```python
from build123d import *

# Parameters (mm, degrees)
SKETCH1_W                  = 100
SKETCH1_H                  = 196.50497
BASE_FLANGE1_DEPTH         = 2.54
CUT_EXTRUDE1_DEPTH         = 221.500917991
CUT_EXTRUDE1_DEPTH_BACK    = 221.500917991
SKETCH1_4_R                = 1.13
SKETCHED_START             = -70.001308696
SKETCHED_BEND3_OUTLINE_R   = 1.13
SKETCHED_BEND3_DEPTH       = 55.325410031
SKETCHED_BEND3_2_DEPTH     = 100
SKETCHED_BEND3_3_DEPTH     = 100
SKETCHED_START_2           = -123
SKETCHED_BEND3_4_OUTLINE_R = 1.13
SKETCHED_BEND3_4_DEPTH     = 4
CUT_EXTRUDE3_DEPTH         = 253.225301809
CUT_EXTRUDE3_DEPTH_BACK    = 253.225301809
SKETCH19_R                 = 1.725
F_4_40_TAPPED_HOLE1_D      = 2.2606


with BuildPart() as part:
    # Base-Flange1: sheet metal written as solids
    # Sketch1 → Base-Flange1 (new body)
    with BuildSketch(Plane.XY):
        with Locations((50, -98.252485)):
            Rectangle(SKETCH1_W, SKETCH1_H)
    extrude(amount=-BASE_FLANGE1_DEPTH)

    # Sketch1<4> → Cut-Extrude1 (cut, two sides: drawn at the far end of the back side and taken through both)
    with BuildSketch(Plane.XY.offset(-CUT_EXTRUDE1_DEPTH_BACK)):
        with Locations((11.9, -6.4268)):
            Circle(SKETCH1_4_R)
        with Locations((88.1, -6.4268)):
            Circle(SKETCH1_4_R)
        with Locations((88.1, -95.3268)):
            Circle(SKETCH1_4_R)
        with Locations((11.9, -95.3268)):
            Circle(SKETCH1_4_R)
    extrude(amount=CUT_EXTRUDE1_DEPTH + CUT_EXTRUDE1_DEPTH_BACK, mode=Mode.SUBTRACT)

    # Sketched Bend3: read off the stored shape, not the designer's step
    # Sketched Bend3 outline → Sketched Bend3 (cut)
    with BuildSketch(Plane(origin=(0, 0, 0), x_dir=(1, 0, 0), z_dir=(0, 0.707106781186549, 0.707106781186546)).offset(SKETCHED_START)):
        with Locations((88.1, -44.309515504)):
            Circle(SKETCHED_BEND3_OUTLINE_R)
        with Locations((11.9, -44.309515504)):
            Circle(SKETCHED_BEND3_OUTLINE_R)
    extrude(amount=SKETCHED_BEND3_DEPTH, mode=Mode.SUBTRACT)

    # Sketched Bend3 2 outline → Sketched Bend3 2 (cut)
    with BuildSketch(Plane.YZ):
        with BuildLine():
            ThreePointArc((-171.665649191, 0), (-169.42029242, -0.446629231), (-167.516770864, -1.718521672))
            Line((-167.516770864, -1.718521672), (-166.695292536, -2.54))
            Line((-166.695292536, -2.54), (0, -2.54))
            Line((0, -2.54), (0, 0))
            Line((0, 0), (-171.665649191, 0))
        make_face()
    extrude(amount=SKETCHED_BEND3_2_DEPTH, mode=Mode.SUBTRACT)

    # Sketched Bend3 3 outline → Sketched Bend3 3 (add)
    with BuildSketch(Plane.YZ):
        with BuildLine():
            Line((-48.542978443, -120.692314093), (-166.695292536, -2.54))
            Line((-166.695292536, -2.54), (-171.665649191, -2.54))
            ThreePointArc((-171.665649191, -2.54), (-170.392308339, -2.793283244), (-169.312822088, -3.514572896))
            Line((-169.312822088, -3.514572896), (-50.339029667, -122.488365317))
            Line((-50.339029667, -122.488365317), (-48.542978443, -120.692314093))
        make_face()
    extrude(amount=SKETCHED_BEND3_3_DEPTH)

    # Sketched Bend3 4 outline → Sketched Bend3 4 (cut)
    with BuildSketch(Plane(origin=(0, 0, 0), x_dir=(1, 0, 0), z_dir=(0, 0.707106781186549, 0.707106781186546)).offset(SKETCHED_START_2)):
        with Locations((11.9, 44.590484496)):
            Circle(SKETCHED_BEND3_4_OUTLINE_R)
        with Locations((88.1, 44.590484496)):
            Circle(SKETCHED_BEND3_4_OUTLINE_R)
        with Locations((88.1, -44.309515504)):
            Circle(SKETCHED_BEND3_4_OUTLINE_R)
        with Locations((11.9, -44.309515504)):
            Circle(SKETCHED_BEND3_4_OUTLINE_R)
    extrude(amount=SKETCHED_BEND3_4_DEPTH, mode=Mode.SUBTRACT)

    # Sketch19 → Cut-Extrude3 (cut, two sides: drawn at the far end of the back side and taken through both)
    with BuildSketch(Plane.XY.offset(-CUT_EXTRUDE3_DEPTH_BACK)):
        with Locations((10, -179.08497)):
            Circle(SKETCH19_R)
        with Locations((50, -179.08497)):
            Circle(SKETCH19_R)
        with Locations((90, -179.08497)):
            Circle(SKETCH19_R)
        with Locations((50, -189.08497)):
            Circle(SKETCH19_R)
        with Locations((90, -189.08497)):
            Circle(SKETCH19_R)
        with Locations((10, -189.08497)):
            Circle(SKETCH19_R)
    extrude(amount=CUT_EXTRUDE3_DEPTH + CUT_EXTRUDE3_DEPTH_BACK, mode=Mode.SUBTRACT)

    # #4-40 Tapped Hole1 (through all)
    with Locations(Plane(origin=(88.1, -115.949205151, -53.286087384), x_dir=(0, -0.707106781187, 0.707106781187), z_dir=(0, 0.707106781187, 0.707106781187))):
        with Locations((0, 0), (0, -76.2), (-88.9, -76.2), (-88.9, 0)):
            Hole(F_4_40_TAPPED_HOLE1_D / 2)


solid = part.part
```
Work out the finished part from the listing and answer in its coordinate system (mm). A direction names the side the tool comes from. Give positions to 0.01 mm unless a question says otherwise; leave off trailing zeros. Write each loop counter-clockwise with the first axis right and the second up, starting at its lowest first coordinate (ties: lowest second). Pieces come first, ordered by that corner, then holes.
(1) Straight lines are drawn through the part: line 1 (Y direction, x = 90, z = -1.75); line 2 (Y direction, x = 50, z = -1.25); line 3 (Z direction, x = 60, y = -173.5). For each, find the intervals that lie inside material, in ascending order.
Final values:
line 1: y = -196.5 to -190.81, -187.36 to -180.81, -177.36 to -167.49
line 2: y = -196.5 to -190.81, -187.36 to -180.81, -177.36 to -168.05
line 3: z = -2.54 to 0
(2) The part is cut by section C-C on z = -69. Write down the section's boundary in (x, y).
Final values:
outline: (0, -103.83) - (100, -103.83) - (100, -100.24) - (0, -100.24) - close
(3) The part is cut by section B-B on y = -137.5. Write down the section's boundary in (x, z).
Final values:
outline: (0, -35.33) - (100, -35.33) - (100, -31.74) - (0, -31.74) - close
(4) Which of the six approach directions +Z, -Z, +X, -X, +Y, -Y give full straight-line access (tool end or side, diameter ignored) to faces 1 (the flat face through (49, -184, -2.54)), 2 (the flat face through (49.3, -107.197, -62.038))?
Final values:
face 1: -Z, +X, -X, -Y
face 2: +Z, +X, -X, +Y
(5) Flat-ended cylindrical pins translate along their axes: pin 1 Ø5.5 at (x, y) = (90, -179.08) entering from -Z; pin 2 Ø3 at (x, y) = (48.5, -156.5) entering from -Z; pin 3 Ø20 at (x, y) = (25.5, -180.5) entering from -Z. Find the tip coordinate at first contact, or state that the pin passes through.
Final values:
pin 1: stops at z = -2.54
pin 2: stops at z = -17.83
pin 3: stops at z = -2.75
(6) The mould has two halves that part along X. Classify faces 3 (the flat face through (100, -123, -47)), 4 (the cylindrical face through (49.63, -180.77, -1.29)), 5 (the cylindrical face through (11.212, -54.632, -116.424)), 6 (the flat face through (49, -184, 0)): pulls with the +X half, pulls with the -X half, needs draft (parallel to the pull), parting line crosses it, or undercut.
Final values:
face 3: pulls with the +X half
face 4: undercut
face 5: undercut
face 6: needs draft
(7) The part is cut by section A-A on x = 64.5. Write down the section's boundary in (y, z).
Final values:
outline: (-196.5, -2.54) - (-171.67, -2.54) arc R3.33 cw to (-169.31, -3.51) - (-50.34, -122.49) - (-48.54, -120.69) - (-167.52, -1.72) arc R5.87 ccw to (-171.67, 0) - (-196.5, 0) - close
